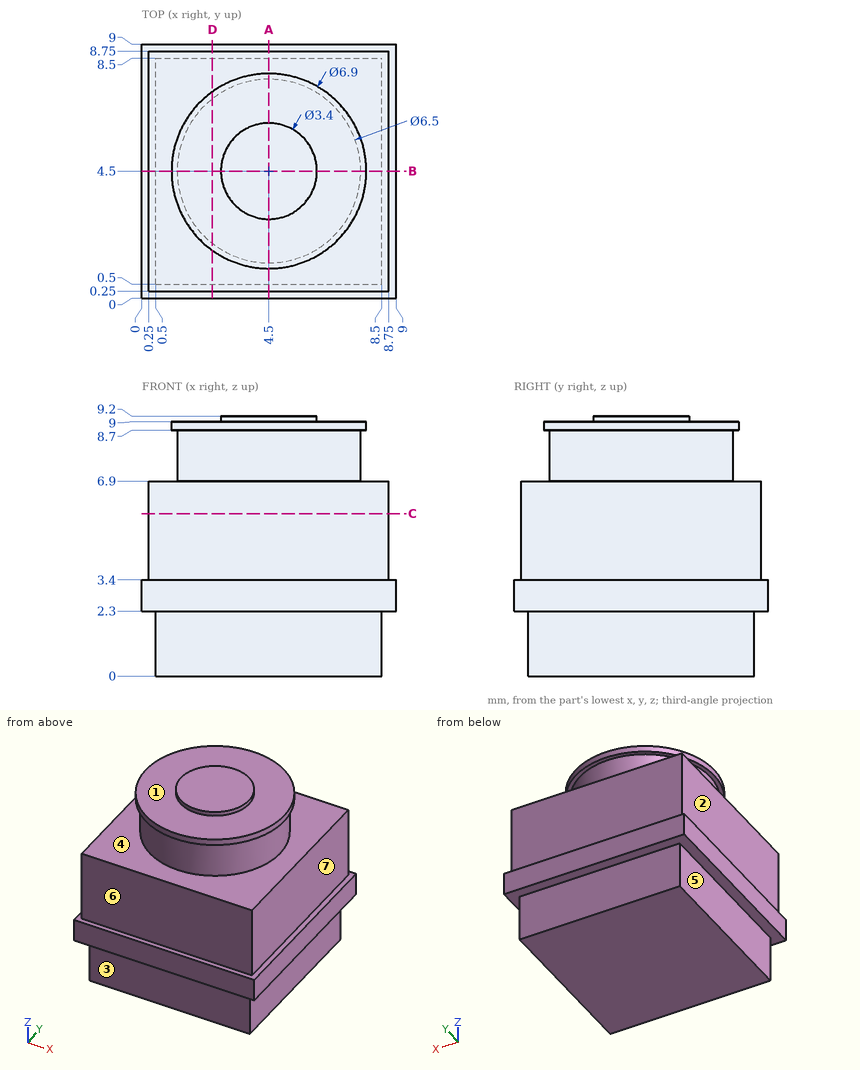
The drawing under review shows one solid part. Ordinate dimensions are in mm from its lowest x, y, z. A direction names the side the tool comes from. Coordinates: 2 decimals unless noted, no trailing zeros. Loops run counter-clockwise (first coordinate to the right, second up) from the corner with the lowest first, then second, coordinate; pieces in that order, holes last.
Item 1: Add section C-C (z = 5.75). Write out the cut boundary in (x, y), and give its area (4 significant figures).
Completed:
outline: (0.25, 0.25) - (8.75, 0.25) - (8.75, 8.75) - (0.25, 8.75) - close
area: 72.25 mm2
Item 2: Add section D-D (x = 2.5). Write out the cut boundary in (y, z), and give its area (3 significant figures).
Completed:
outline: (0, 2.3) - (0.5, 2.3) - (0.5, 0) - (8.5, 0) - (8.5, 2.3) - (9, 2.3) - (9, 3.4) - (8.75, 3.4) - (8.75, 6.9) - (7.06, 6.9) - (7.06, 8.7) - (7.31, 8.7) - (7.31, 9) - (1.69, 9) - (1.69, 8.7) - (1.94, 8.7) - (1.94, 6.9) - (0.25, 6.9) - (0.25, 3.4) - (0, 3.4) - close
area: 69.0 mm2
Item 3: For the marked faces 1, 2, 3 and 4, list the 3-axis set-ups (+Z, -Z, +X, -X, +Y, -Y) from which the entire face can be reached by the end or side of a thin tool; tool diameter is ignored.
Completed:
face 1: +Z
face 2: +Z, -X, +Y, -Y
face 3: -Z, +X, -X, -Y
face 4: none
Item 4: Draft analysis for pull direction X (two halves, no side actions). For the marked faces 5, 6 and 7, state which applies: pulls with the +X half, pulls with the -X half, needs draft (parallel to the pull), parting line crosses it, or undercut.
Completed:
face 5: pulls with the -X half
face 6: needs draft
face 7: pulls with the +X half
Item 5: Add section A-A (x = 4.5). Write out the cut boundary in (y, z).
Completed:
outline: (0, 2.3) - (0.5, 2.3) - (0.5, 0) - (8.5, 0) - (8.5, 2.3) - (9, 2.3) - (9, 3.4) - (8.75, 3.4) - (8.75, 6.9) - (7.75, 6.9) - (7.75, 8.7) - (7.95, 8.7) - (7.95, 9) - (6.2, 9) - (6.2, 9.2) - (2.8, 9.2) - (2.8, 9) - (1.05, 9) - (1.05, 8.7) - (1.25, 8.7) - (1.25, 6.9) - (0.25, 6.9) - (0.25, 3.4) - (0, 3.4) - close
Item 6: Clearance check with flat-ended pins moving along their axes: pin 1 (2 mm diameter, centred on x = 6.5, y = 7, fed in from +Z); pin 2 (1.8 mm diameter, centred on y = 4, z = 5, fed in from +X); pin 3 (4 mm diameter, centred on x = 5, y = 6.5, fed in from +Z); pin 4 (1.8 mm diameter, centred on y = 6.5, z = 6, fed in from -X). State where each tip first meets the part, or that it passes through.
Completed:
pin 1: stops at z = 9
pin 2: stops at x = 8.75
pin 3: stops at z = 9.2
pin 4: stops at x = 0.25
Item 7: Wall thickness on L1, parallel to X at y = 3.25, z = 1.75; L2, parallel to Y at x = 3.25, z = 4.5: over which ranges is each line inside the solid? List them lowest first.
Completed:
L1: x = 0.5 to 8.5
L2: y = 0.25 to 8.75
